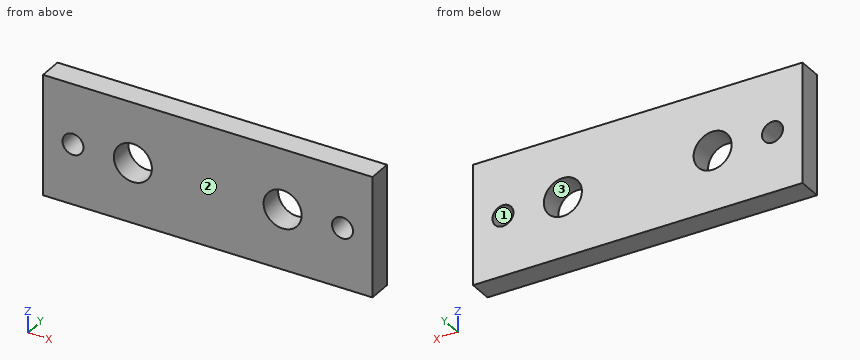
Solid Edge part; units mm, degrees
sketch "Sketch1" plane through (0, 0, 0) normal (0, -1, 0) x (1, 0, 0)
  line L0 (-27.5, 10) -> (27.5, 10)
  line L1 (27.5, 10) -> (27.5, -10)
  line L2 (27.5, -10) -> (-27.5, -10)
  line L3 (-27.5, -10) -> (-27.5, 10)
  dimension "D1" = 27.5
  dimension "D2" = 27.5
extrude "Protrusion1" add sketch "Sketch1" against normal blind 4
hole "Bohrung_1" at (12.5, 0, 0) direction (0, 1, 0) diameter 6.35 end up to next
hole "Hole1" at (-12.5, 0, 0) direction (0, 1, 0) diameter 6.35 end up to next
hole "Bohrung_3" at (22.5, 0, 0) direction (0, 1, 0) diameter 3.5 end up to next
hole "Hole2" at (-22.5, 0, 0) direction (0, 1, 0) diameter 3.5 end up to next
Source: CAD feature listing. Evaluate the final solid. Frame: model axes, mm. Face numbers are marked on the shaded views. Coordinates: 2 decimals unless noted, no trailing zeros. Write each loop counter-clockwise with the first axis right and the second up, starting at its lowest first coordinate (ties: lowest second). Pieces come first, ordered by that corner, then holes. Notation, with made-up numbers: M 3,76.25 L 11,76.25 A18 cw 11,107.25 Z; hole C 32,62 d2. An arc over 180 degrees is marked long. Answer as a JSON object with one key per item and string values.
1. Cut plane C-C on y = 2.35. Output: boundary loops of the cut face in (x, z) (3 decimals).
Evaluation:
{"outline": "M -27.5,-10 L 27.5,-10 L 27.5,10 L -27.5,10 Z; hole C -22.5,0 d3.5; hole C -12.5,0 d6.35; hole C 12.5,0 d6.35; hole C 22.5,0 d3.5"}
2. Ray query, L1, parallel to X at y = 2.85, z = 0 (3 decimals); L2, parallel to Z at x = -22.5, y = 1.75; L3, parallel to Z at x = -12.5, y = 2.45 (3 decimals). Return the intervals inside material, ascending.
Evaluation:
{"L1": "-27.5 to -24.25, -20.75 to -15.675, -9.325 to 9.325, 15.675 to 20.75, 24.25 to 27.5", "L2": "-10 to -1.75, 1.75 to 10", "L3": "-10 to -3.175, 3.175 to 10"}
3. Cut plane D-D on z = 2.5. Output: boundary loops of the cut face in (x, y), plus the area to 3 significant figures.
Evaluation:
{"outline": "M -27.5,0 L -14.46,0 L -14.46,4 L -27.5,4 Z; M -10.54,0 L 10.54,0 L 10.54,4 L -10.54,4 Z; M 14.46,0 L 27.5,0 L 27.5,4 L 14.46,4 Z", "area": "189 mm^2"}
4. Cut plane A-A on x = -22.5. Output: boundary loops of the cut face in (y, z), plus the area to 3 significant figures.
Evaluation:
{"outline": "M 0,-10 L 4,-10 L 4,-1.75 L 0,-1.75 Z; M 0,1.75 L 4,1.75 L 4,10 L 0,10 Z", "area": "66.0 mm^2"}
5. Cut plane B-B on z = 0. Output: boundary loops of the cut face in (x, y) (3 decimals).
Evaluation:
{"outline": "M -27.5,0 L -24.25,0 L -24.25,4 L -27.5,4 Z; M -20.75,0 L -15.675,0 L -15.675,4 L -20.75,4 Z; M -9.325,0 L 9.325,0 L 9.325,4 L -9.325,4 Z; M 15.675,0 L 20.75,0 L 20.75,4 L 15.675,4 Z; M 24.25,0 L 27.5,0 L 27.5,4 L 24.25,4 Z"}
6. Draft query along X for the marked faces 1, 2 and 3. Return one class per face: released by +X, released by -X, zero draft, split by the parting line, or undercut.
Evaluation:
{"face 1": "undercut", "face 2": "zero draft", "face 3": "undercut"}
